Part model, mm, in its own coordinate system. A direction names the side the tool comes from. Give positions to 0.01 mm unless a question says otherwise; leave off trailing zeros. Write each loop counter-clockwise with the first axis right and the second up, starting at its lowest first coordinate (ties: lowest second). Pieces come first, ordered by that corner, then holes. Notation, with made-up numbers: M 41.25,30.25 L 100.25,30.25 A25 cw 100.25,65.25 Z; hole C 52.5,49.5 d6. An arc over 180 degrees is marked long. Write item = value, one per line. Start each with the question number.
from build123d import *

# Parameters (mm, degrees)
F1_DEPTH = 30
F2_DEPTH = 20
F3_DEPTH = 10


with BuildPart() as f1:
    # F0 (on Top) → F1 (new body)
    with BuildSketch(Plane.XY):
        Polygon((10, 15), (0, 0), (30, 0), (20, 15), align=None)
        Polygon((0, 30), (0, 0), (10, 15), align=None)
        Polygon((20, 15), (30, 0), (30, 30), align=None)
        Polygon((30, 30), (0, 30), (10, 15), (20, 15), align=None)
    extrude(amount=-F1_DEPTH)

    # F0 (on Top) → F2 (cut)
    with BuildSketch(Plane.XY):
        Polygon((10, 15), (0, 0), (30, 0), (20, 15), align=None)
    extrude(amount=-F2_DEPTH, mode=Mode.SUBTRACT)

    # F0 (on Top) → F3 (cut)
    with BuildSketch(Plane.XY):
        Polygon((0, 30), (0, 0), (10, 15), align=None)
        Polygon((20, 15), (30, 0), (30, 30), align=None)
    extrude(amount=-F3_DEPTH, mode=Mode.SUBTRACT)


solid = f1.part
Q1. Slice it at C-C (y = 7.25). Give the cut face in (x, z), and give its area (3 significant figures).
Q2. Probe line 1 along Z through (x, y) = (14.5, 8); line 2 along X through (y, z) = (6.5, -15.75); line 3 along Z through (x, y) = (22.5, 16.75). List the from-to ranges inside material, lowest first.
Q3. Slice it at D-D (y = 21). Give the cut face in (x, z).
Q4. Two-plate mould, pull along X, no slides. Class faces 1 (the face through (15, 15, -10)), 2 (the face through (5.07, 22.395, -4.93)), 3 (the face through (15, 0, -25)): +X half, -X half, draft (parallel to the pull), parting line (faces both ways), or undercut.
Q5. Tool access for faces 4 (the face through (5.07, 7.605, -14.93)), 5 (the face through (25.07, 22.605, -4.93)), 6 (the face through (15, 30, -15)), 7 (the face through (4, 15, -10)): list every direction of +Z, -Z, +X, -X, +Y, -Y with a clear straight run to the whole face (end or side of a thin tool).
Q6. Slice it at A-A (z = -16.5). Give the cut face in (x, y).
Q7. Drop flat-ended pins along their axis: P1, Ø12, axis at x = 9, y = 4.5, coming from the +Z side; P2, Ø12, axis at x = 8, z = -13.5, coming from the -Y side; P3, Ø2, axis at y = 18.5, z = -7.5, coming from the +X side. Give the stop position or say it passes through.
Q8. Slice it at B-B (x = 17). Give the cut face in (y, z).
Working result:
q1.outline = M 0,-30 L 30,-30 L 30,-10 L 25.17,-10 L 25.17,-20 L 4.83,-20 L 4.83,-10 L 0,-10 Z
q1.area = 397 mm2
q2.line_1 = -30 to -20
q2.line_2 = 0 to 4.33, 25.67 to 30
q2.line_3 = -30 to -10
q3.outline = M 0,-30 L 30,-30 L 30,-10 L 24,-10 L 24,0 L 6,0 L 6,-10 L 0,-10 Z
q4.face_1 = undercut
q4.face_2 = -X half
q4.face_3 = draft
q5.face_4 = +Z, -Y
q5.face_5 = +Z, +X, -Y
q5.face_6 = +Z, -Z, +X, -X, +Y
q5.face_7 = +Z, -X, -Y
q6.outline = M 0,0 L 10,15 L 20,15 L 30,0 L 30,30 L 0,30 Z
q7.P1 = -10
q7.P2 = 3
q7.P3 = 23
q8.outline = M 0,-30 L 30,-30 L 30,0 L 15,0 L 15,-20 L 0,-20 Z
